Build history of the part. All positions in model axes, mm. A direction names the side the tool comes from. Give positions to 0.01 mm unless a question says otherwise; leave off trailing zeros. Loops run counter-clockwise (first coordinate to the right, second up) from the corner with the lowest first, then second, coordinate; pieces in that order, holes last. Notation, with made-up numbers: (-37, 76.25) - (-3, 76.25) arc R21 ccw to (-3, 100.25) - close; hole circle Ø7 at (51, 4.5). An arc over 180 degrees is marked (long way). Return JSON: item names as keys, results as strings. Group by question number.
1) Drill centre lines: probe 1 along X at (y, z) = (9.7, -169.5) (3 decimals); probe 2 along X at (y, z) = (-9.3, 142) (3 decimals); probe 3 along Y at (x, z) = (5.5, 2). Where is each one in solid material? Low to high. Write a range as from..to.
2) Slice it at A-A (z = -151). List the corners of the cut face in (x, y).
3) Mould opens along Z. For faces 1 (the face through (-0.521, 9.507, -145.966)), 2 (the face through (-0.8, -9.6, 200)), 3 (the face through (9, 0, 3)) say: released by +Z, released by -Z, zero draft, split by the parting line, or undercut.
4) Drop flat-ended pins along their axis: pin 1 (2.5 mm diameter, centred on x = -1, z = 189.5, fed in from -Y); pin 2 (7 mm diameter, centred on x = 0, z = 142, fed in from +Y); pin 3 (4.5 mm diameter, centred on y = 0, z = 19, fed in from +X). Give the stop position or say it passes through.
5) 3-axis set-ups, long thin cutter, end or side, ignore diameter. For faces 4 (the face through (0, -9, 3)), 5 (the face through (-0.521, 9.507, 123.034)), 6 (the face through (0, -10, 3)), 7 (the face through (0, 10, 3)), 8 (the face through (9.5, -2.4, 22.2)): which of +Z, -Z, +X, -X, +Y, -Y reach the whole face in a straight line?
```python
from build123d import *

# Parameters (mm, degrees)
SKETCH_1_W               = 20
SKETCH_1_H               = 20
EXTRUDE_1_DEPTH          = 200
SKETCH_2_W               = 18
SKETCH_2_H               = 18
CUT_EXTRUDE_1_DEPTH      = 201
CUT_EXTRUDE_1_DEPTH_BACK = 201
CUT_EXTRUDE_START        = -21
SKETCH_3_R               = 1.525
CUT_EXTRUDE_2_DEPTH      = 22
SKETCH_4_R               = 2.025
CUT_EXTRUDE_3_DEPTH      = 21
SKETCH_5_R               = 4
CUT_EXTRUDE_4_DEPTH      = 1
SKETCH_6_R               = 1.525
CUT_EXTRUDE_5_DEPTH      = 22
SKETCH_7_R               = 2.025
CUT_EXTRUDE_6_DEPTH      = 1
CUT_EXTRUDE_6_DEPTH_BACK = 21
SKETCH_8_R               = 4
CUT_EXTRUDE_7_DEPTH      = 3
CUT_EXTRUDE_8_DEPTH      = 1
CUT_EXTRUDE_8_DEPTH_BACK = 21


with BuildPart() as part:
    # 草图1 → 凸台-拉伸1 (new body, symmetric)
    with BuildSketch(Plane.XY):
        Rectangle(SKETCH_1_W, SKETCH_1_H)
    extrude(amount=EXTRUDE_1_DEPTH, both=True)

    # 草图2 → 切除-拉伸1 (cut, two sides)
    with BuildSketch(Plane.XY) as cut_extrude_1_sk:
        Rectangle(SKETCH_2_W, SKETCH_2_H)
    extrude(amount=CUT_EXTRUDE_1_DEPTH, mode=Mode.SUBTRACT)
    extrude(cut_extrude_1_sk.sketch, amount=-CUT_EXTRUDE_1_DEPTH_BACK, mode=Mode.SUBTRACT)

    # 草图3 → 切除-拉伸2 (cut)
    with BuildSketch(Plane(origin=(0, 10, 0), x_dir=(1, 0, 0), z_dir=(0, 1, 0)).offset(CUT_EXTRUDE_START)):
        with Locations((-1, -189.5)):
            Circle(SKETCH_3_R)
        with Locations((-1, -169.5)):
            Circle(SKETCH_3_R)
    cut_extrude_2 = extrude(amount=CUT_EXTRUDE_2_DEPTH, mode=Mode.SUBTRACT)

    # 镜向1: 切除-拉伸2 across plane
    add(cut_extrude_2.mirror(Plane.XY), mode=Mode.SUBTRACT)

    # 草图4 → 切除-拉伸3 (cut, through all)
    with BuildSketch(Plane(origin=(10, 0, 0), x_dir=(0, 0, -1), z_dir=(1, 0, 0))):
        with Locations((-19, 0)):
            Circle(SKETCH_4_R)
        with Locations((19, 0)):
            Circle(SKETCH_4_R)
    extrude(amount=-CUT_EXTRUDE_3_DEPTH, mode=Mode.SUBTRACT)

    # 草图5 → 切除-拉伸4 (cut)
    with BuildSketch(Plane(origin=(10, 0, 0), x_dir=(0, 0, -1), z_dir=(1, 0, 0))):
        with Locations((-19, 0)):
            Circle(SKETCH_5_R)
        with Locations((19, 0)):
            Circle(SKETCH_5_R)
    extrude(amount=-CUT_EXTRUDE_4_DEPTH, mode=Mode.SUBTRACT)

    # 草图6 → 切除-拉伸5 (cut)
    with BuildSketch(Plane(origin=(10, 0, 0), x_dir=(0, 0, -1), z_dir=(1, 0, 0)).offset(CUT_EXTRUDE_START)):
        with Locations((159.5, 6)):
            Circle(SKETCH_6_R)
        with Locations((179.5, 6)):
            Circle(SKETCH_6_R)
    cut_extrude_5 = extrude(amount=CUT_EXTRUDE_5_DEPTH, mode=Mode.SUBTRACT)

    # 草图7 → 切除-拉伸6 (cut, two sides)
    with BuildSketch(Plane(origin=(0, 10, 0), x_dir=(1, 0, 0), z_dir=(0, 1, 0))) as cut_extrude_6_sk:
        with Locations((0, 142)):
            Circle(SKETCH_7_R)
        with Locations((0, 127)):
            Circle(SKETCH_7_R)
        with Locations((0, -127)):
            Circle(SKETCH_7_R)
        with Locations((0, -142)):
            Circle(SKETCH_7_R)
    extrude(amount=CUT_EXTRUDE_6_DEPTH, mode=Mode.SUBTRACT)
    extrude(cut_extrude_6_sk.sketch, amount=-CUT_EXTRUDE_6_DEPTH_BACK, mode=Mode.SUBTRACT)

    # 草图8 → 切除-拉伸7 (cut)
    with BuildSketch(Plane(origin=(0, 10, 0), x_dir=(1, 0, 0), z_dir=(0, 1, 0))):
        with Locations((0, 142)):
            Circle(SKETCH_8_R)
        with Locations((0, 127)):
            Circle(SKETCH_8_R)
        with Locations((0, -127)):
            Circle(SKETCH_8_R)
        with Locations((0, -142)):
            Circle(SKETCH_8_R)
    extrude(amount=-CUT_EXTRUDE_7_DEPTH, mode=Mode.SUBTRACT)

    # 镜向2: 切除-拉伸5 across plane
    add(cut_extrude_5.mirror(Plane.XY), mode=Mode.SUBTRACT)

    # 草图9 → 切除-拉伸8 (cut, two sides)
    with BuildSketch(Plane(origin=(0, 10, 0), x_dir=(1, 0, 0), z_dir=(0, 1, 0))) as cut_extrude_8_sk:
        with BuildLine():
            Line((4, 85), (4, 55))
            ThreePointArc((4, 55), (0, 51), (-4, 55))
            Line((-4, 55), (-4, 85))
            ThreePointArc((-4, 85), (0, 89), (4, 85))
        make_face()
        with BuildLine():
            Line((4, -85), (4, -55))
            ThreePointArc((4, -55), (0, -51), (-4, -55))
            Line((-4, -55), (-4, -85))
            ThreePointArc((-4, -85), (0, -89), (4, -85))
        make_face()
    extrude(amount=CUT_EXTRUDE_8_DEPTH, mode=Mode.SUBTRACT)
    extrude(cut_extrude_8_sk.sketch, amount=-CUT_EXTRUDE_8_DEPTH_BACK, mode=Mode.SUBTRACT)


solid = part.part
```
Results:
{
 "1": {"probe 1": "-10..-2.525, 0.525..10", "probe 2": "-10..-2.025, 2.025..10", "probe 3": "-10..-9, 9..10"},
 "2": {"outline": "(-10, -10) - (10, -10) - (10, 10) - (-10, 10) - close; hole (-9, -9) - (9, -9) - (9, 9) - (-9, 9) - close"},
 "3": {"face 1": "undercut", "face 2": "released by +Z", "face 3": "zero draft"},
 "4": {"pin 1": "through", "pin 2": "y = -9", "pin 3": "x = -9"},
 "5": {"face 4": "+Z, -Z", "face 5": "+Y", "face 6": "+Z, -Z, +X, -X, -Y", "face 7": "+Z, -Z, +X, -X, +Y", "face 8": "+X"}
}
